The listing builds one solid part. Answer for the finished solid, in the listing's coordinates (mm). Round coordinates to 2 decimals unless told otherwise and drop trailing zeros. Loops run counter-clockwise (first coordinate to the right, second up) from the corner with the lowest first, then second, coordinate; pieces in that order, holes last. Notation, with made-up numbers: (10, -1) - (57, -1) arc R6 cw to (57, 9) - close; hole circle Ø3 at (68, 48). An arc over 180 degrees is marked (long way). One line per item, written item: value.
```python
from build123d import *

# Parameters (mm, degrees)
SKETCH_W          = 20
SKETCH_H          = 120
PAD_DEPTH         = 5
SKETCH001_W       = 15.635981
SKETCH001_H       = 23
POCKET_DEPTH      = 5.001
SKETCH002_W       = 5
SKETCH002_H       = 31
PAD001_DEPTH      = 15
PAD001_DEPTH_BACK = 25
POCKET001_DEPTH   = 5
CHAMFER_SIZE      = 5


with BuildPart() as part:
    # Sketch → Pad (new body)
    with BuildSketch(Plane.XY):
        with Locations((0, 60)):
            Rectangle(SKETCH_W, SKETCH_H)
    extrude(amount=PAD_DEPTH)

    # Sketch001 → Pocket (cut, through all)
    with BuildSketch(Plane.XY.offset(5)):
        with BuildLine():
            ThreePointArc((-4, 11.8), (-6.8, 9), (-4, 6.2))
            Line((-4, 6.2), (4, 6.2))
            ThreePointArc((4, 6.2), (6.8, 9), (4, 11.8))
            Line((-4, 11.8), (4, 11.8))
        make_face()
        with BuildLine():
            ThreePointArc((-4, 21.8), (-6.8, 19), (-4, 16.2))
            Line((-4, 16.2), (4, 16.2))
            ThreePointArc((4, 16.2), (6.8, 19), (4, 21.8))
            Line((-4, 21.8), (4, 21.8))
        make_face()
        with Locations((2.81799, 108.532179)):
            Rectangle(SKETCH001_W, SKETCH001_H)
        with BuildLine():
            ThreePointArc((-4.113055, 31.8), (-6.913055, 29), (-4.113055, 26.2))
            Line((-4.113055, 26.2), (4.113055, 26.2))
            ThreePointArc((4.113055, 26.2), (6.913055, 29), (4.113055, 31.8))
            Line((-4.113055, 31.8), (4.113055, 31.8))
        make_face()
    extrude(amount=-POCKET_DEPTH, mode=Mode.SUBTRACT)

    # Sketch002 → Pad001 (new body, two sides)
    with BuildSketch(Plane.XY.offset(5)) as pad001_sk:
        with Locations((-7.5, 104.5)):
            Rectangle(SKETCH002_W, SKETCH002_H)
    extrude(amount=PAD001_DEPTH)
    extrude(pad001_sk.sketch, amount=-PAD001_DEPTH_BACK)

    # Sketch003 → Pocket001 (cut)
    with BuildSketch(Plane.YZ.offset(-5)):
        with BuildLine():
            ThreePointArc((116.657567, 15), (114.857567, 16.8), (113.057567, 15))
            Line((113.057567, 15), (113.057567, -15))
            ThreePointArc((113.057567, -15), (114.857567, -16.8), (116.657567, -15))
            Line((116.657567, 15), (116.657567, -15))
        make_face()
        with BuildLine():
            ThreePointArc((106.657567, 15), (104.857567, 16.8), (103.057567, 15))
            Line((103.057567, 15), (103.057567, -15))
            ThreePointArc((103.057567, -15), (104.857567, -16.8), (106.657567, -15))
            Line((106.657567, 15), (106.657567, -15))
        make_face()
        Polygon((88, 5), (103, 21), (88, 21), align=None)
        Polygon((88, 0), (103, -21), (88, -21), align=None)
    extrude(amount=-POCKET001_DEPTH, mode=Mode.SUBTRACT)

    # Chamfer
    chamfer_edges = [part.edges().sort_by_distance(p)[0] for p in [
        (10, 0, 2.5),
        (10, 97.032179, 2.5),
        (-7.5, 120, 20),
        (-7.5, 120, -20),
    ]]
    chamfer(chamfer_edges, length=CHAMFER_SIZE)


solid = part.part
```
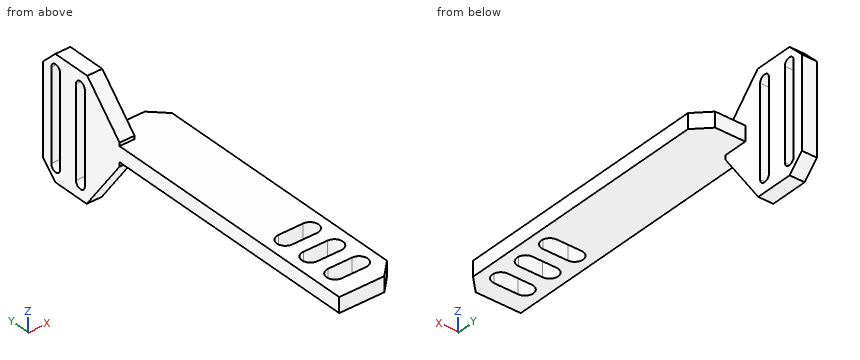
1) A cutting plane is placed at D-D on x = 8. Give the vertices of the cut face in (y, z).
Final values:
outline: (3, 0) - (94.03, 0) - (94.03, 5) - (3, 5) - close
2) Consider L1, parallel to Y at x = -7.5, z = -15; L2, parallel to Y at x = -9, z = 8; L3, parallel to Z at x = 7, y = 91. Determine where each line is inside the solid, lowest interval first.
Final values:
L1: 98.71 to 103.06, 106.66 to 113.06, 116.66 to 120
L2: 90.81 to 103.06, 106.66 to 113.06, 116.66 to 120
L3: 0 to 5
3) Each of these flat-tipped pins is pushed along its axis until it touches: pin 1 Ø1 at (x, z) = (-6, 7) entering from -Y; pin 2 Ø10 at (x, y) = (0.5, 43) entering from +Z; pin 3 Ø12 at (x, y) = (6.5, 68.5) entering from -Z; pin 4 Ø12 at (y, z) = (50.5, 11.5) entering from -X. Where does it stop, or does it pass through?
Final values:
pin 1: y = 89.41
pin 2: z = 5
pin 3: z = 0
pin 4: through
4) A cutting plane is placed at B-B on z = -8.5. Give the vertices of the cut face in (x, y).
Final values:
outline: (-10, 94.07) - (-5, 94.07) - (-5, 103.06) - (-10, 103.06) - close; (-10, 106.66) - (-5, 106.66) - (-5, 113.06) - (-10, 113.06) - close; (-10, 116.66) - (-5, 116.66) - (-5, 120) - (-10, 120) - close
5) A cutting plane is placed at A-A on y = 29. Give the vertices of the cut face in (x, z).
Final values:
outline: (-10, 0) - (-6.91, 0) - (-6.91, 5) - (-10, 5) - close; (6.91, 0) - (10, 0) - (10, 5) - (6.91, 5) - close
6) A cutting plane is placed at C-C on y = 48. Give the vertices of the cut face in (x, z), and give its area (3 significant figures).
Final values:
outline: (-10, 0) - (10, 0) - (10, 5) - (-10, 5) - close
area: 100 mm2
